CAD build for the part. Positions are in the model's coordinates, mm. Face numbers are marked on the shaded views. A direction names the side the tool comes from. Round coordinates to 2 decimals unless told otherwise and drop trailing zeros. Loops run counter-clockwise (first coordinate to the right, second up) from the corner with the lowest first, then second, coordinate; pieces in that order, holes last. Notation, with made-up numbers: (85, 29) - (105, 29) arc R10 ccw to (105, 37) - close; hole circle Ø5 at (-17.5, 20.5). An arc over 180 degrees is marked (long way). One line per question, with ' | ' between items.
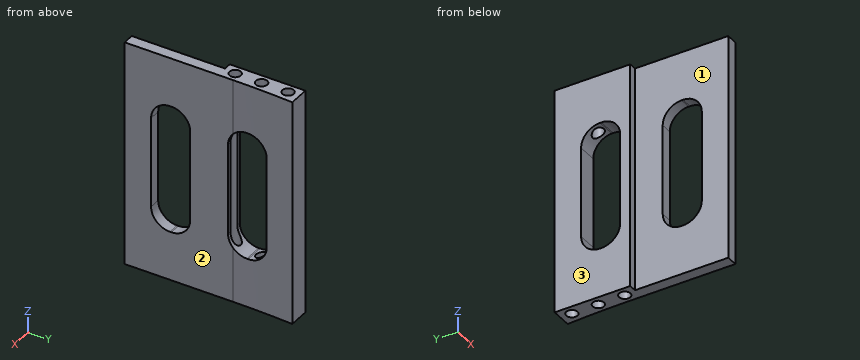
```python
from build123d import *

# Parameters (mm, degrees)
RESSALTO_EXTRUS_O1_DEPTH = 60
ESBO_O7_R                = 2.076684074
CORTE_EXTRUS_O5_DEPTH    = 61
ESBO_O8_W                = 84.528747457
ESBO_O8_H                = 37.806532702
CORTE_EXTRUS_O6_DEPTH    = 61
ESBO_O9_W                = 39.370764713
ESBO_O9_H                = 9.06161947
CORTE_EXTRUS_O7_DEPTH    = 61
ESBO_O10_W               = 32.42010131
ESBO_O10_H               = 62.029224545
CORTE_EXTRUS_O8_DEPTH    = 61
ESBO_O12_W               = 17.69499929
ESBO_O12_H               = 9
CORTE_EXTRUS_O10_DEPTH   = 61
ESBO_O13_W               = 2
ESBO_O13_H               = 24.699383264
CORTE_EXTRUS_O11_DEPTH   = 61
CORTE_EXTRUS_O12_DEPTH   = 6.517415369
ESBO_O15_R               = 1.5
CORTE_EXTRUS_O13_DEPTH   = 61.0000001


with BuildPart() as part:
    # Esboço1 → Ressalto-extrusão1 (new body)
    with BuildSketch(Plane.XY):
        with BuildLine():
            Line((13.569146061, 27.715579822), (13.569146061, 56.338894978))
            ThreePointArc((13.569146061, 56.338894978), (13.884544414, 68.892766914), (14.829943665, 81.414963086))
            ThreePointArc((14.829943665, 81.414963086), (11.193742071, 116.066691762), (-16.576524471, 95.024435265))
            Line((-16.576524471, 95.024435265), (-16.487894969, 94.437265709))
            Line((-16.487894969, 94.437265709), (-16.369382775, 93.652123615))
            ThreePointArc((-16.369382775, 93.652123615), (-14.270188159, 75.047972701), (-13.569146061, 56.338894978))
            Line((-13.569146061, 56.338894978), (-13.569146061, 27.715579822))
            ThreePointArc((-13.569146061, 27.715579822), (0, 21.02683783), (13.569146061, 27.715579822))
        make_face()
    extrude(amount=RESSALTO_EXTRUS_O1_DEPTH)

    # Esboço7 → Corte-extrusão5 (cut, through all)
    with BuildSketch(Plane(origin=(0, 0, 0), x_dir=(-1, 0, 0), z_dir=(0, 0, -1))):
        with Locations((-0.267564972, 95.19)):
            Circle(ESBO_O7_R)
    extrude(amount=-CORTE_EXTRUS_O5_DEPTH, mode=Mode.SUBTRACT)

    # Esboço8 → Corte-extrusão6 (cut, through all)
    with BuildSketch(Plane.XY.offset(60)):
        with Locations((-3.694100087, 100.318229437)):
            Rectangle(ESBO_O8_W, ESBO_O8_H)
    extrude(amount=-CORTE_EXTRUS_O6_DEPTH, mode=Mode.SUBTRACT)

    # Esboço9 → Corte-extrusão7 (cut, through all)
    with BuildSketch(Plane.XY.offset(60)):
        with Locations((-6.116236296, 23.184770087)):
            Rectangle(ESBO_O9_W, ESBO_O9_H)
    extrude(amount=-CORTE_EXTRUS_O7_DEPTH, mode=Mode.SUBTRACT)

    # Esboço10 → Corte-extrusão8 (cut, through all)
    with BuildSketch(Plane.XY.offset(60)):
        with Locations((-7.640904594, 58.730192094)):
            Rectangle(ESBO_O10_W, ESBO_O10_H)
    extrude(amount=-CORTE_EXTRUS_O8_DEPTH, mode=Mode.SUBTRACT)

    # Esboço12 → Corte-extrusão10 (cut, through all)
    with BuildSketch(Plane.XY.offset(60)):
        with Locations((10.676364632, 76.914963086)):
            Rectangle(ESBO_O12_W, ESBO_O12_H)
    extrude(amount=-CORTE_EXTRUS_O10_DEPTH, mode=Mode.SUBTRACT)

    # Esboço13 → Corte-extrusão11 (cut, through all)
    with BuildSketch(Plane.XY.offset(60)):
        with Locations((9.569146061, 40.065271454)):
            Rectangle(ESBO_O13_W, ESBO_O13_H)
    extrude(amount=-CORTE_EXTRUS_O11_DEPTH, mode=Mode.SUBTRACT)

    # Esboço14 → Corte-extrusão12 (cut, through all)
    with BuildSketch(Plane.ZY.offset(-8.569146061)):
        with BuildLine():
            Line((42, 55.065579822), (18, 55.065579822))
            ThreePointArc((18, 55.065579822), (14.464466094, 56.530045916), (13, 60.065579822))
            Line((13, 60.065579822), (13, 60.414963086))
            ThreePointArc((13, 60.414963086), (14.464466094, 63.950496992), (18, 65.414963086))
            Line((18, 65.414963086), (42, 65.414963086))
            ThreePointArc((42, 65.414963086), (45.535533906, 63.950496992), (47, 60.414963086))
            Line((47, 60.414963086), (47, 60.065579822))
            ThreePointArc((47, 60.065579822), (45.535533906, 56.530045916), (42, 55.065579822))
        make_face()
        with BuildLine():
            Line((42, 34.715579822), (18, 34.715579822))
            ThreePointArc((18, 34.715579822), (14.464466094, 36.180045916), (13, 39.715579822))
            Line((13, 39.715579822), (13, 40.065579822))
            ThreePointArc((13, 40.065579822), (14.464466094, 43.601113728), (18, 45.065579822))
            Line((18, 45.065579822), (42, 45.065579822))
            ThreePointArc((42, 45.065579822), (45.535533906, 43.601113728), (47, 40.065579822))
            Line((47, 40.065579822), (47, 39.715579822))
            ThreePointArc((47, 39.715579822), (45.535533906, 36.180045916), (42, 34.715579822))
        make_face()
    extrude(amount=-CORTE_EXTRUS_O12_DEPTH, mode=Mode.SUBTRACT)

    # Esboço15 → Corte-extrusão13 (cut, through all)
    with BuildSketch(Plane.XY.offset(60)):
        with Locations((11.069146061, 69.414963086)):
            Circle(ESBO_O15_R)
        with Locations((11.069146061, 62.414963086)):
            Circle(ESBO_O15_R)
        with Locations((11.069146061, 55.414963086)):
            Circle(ESBO_O15_R)
    extrude(amount=-CORTE_EXTRUS_O13_DEPTH, mode=Mode.SUBTRACT)


solid = part.part
```
(1) Cut at D-D, the plane x = 11.45. State how many separate pieces and enclosed holes the cut face has, then the cut area to 3 significant figures.
Results found:
separate pieces: 5 | enclosed holes: 1 | area: 1,650 mm²
(2) Cut at C-C, the plane z = 7. Write the cut outline in (x, y).
Results found:
outline: (8.57, 52.41) - (10.57, 52.41) - (10.57, 27.72) - (13.57, 27.72) - (13.57, 56.34) arc R250 cw to (14.09, 72.41) - (8.57, 72.41) - close; hole circle Ø3 at (11.07, 55.41); hole circle Ø3 at (11.07, 62.41); hole circle Ø3 at (11.07, 69.41)
(3) Cut at B-B, the plane y = 43. Write the cut outline in (x, z), then the cut area to 3 significant figures.
Results found:
outline: (10.57, 0) - (13.57, 0) - (13.57, 13.95) - (10.57, 13.95) - close; (10.57, 46.05) - (13.57, 46.05) - (13.57, 60) - (10.57, 60) - close | area: 83.7 mm²
(4) Cut at A-A, the plane z = 15.5. Write the cut outline in (x, y).
Results found:
outline: (8.57, 52.41) - (10.57, 52.41) - (10.57, 44.4) - (13.57, 44.4) - (13.57, 55.74) - (12.53, 55.74) arc R1.5 cw (long way) to (9.6, 55.74) - (8.57, 55.74) - close; (8.57, 64.75) - (13.71, 64.75) arc R250 cw to (14.09, 72.41) - (8.57, 72.41) - close; (10.57, 27.72) - (13.57, 27.72) - (13.57, 35.39) - (10.57, 35.39) - close; hole circle Ø3 at (11.07, 69.41)
(5) Tool access for the marked faces 1, 2 and 3: list every direction of +Z, -Z, +X, -X, +Y, -Y with a clear straight run to the whole face (end or side of a thin tool).
Results found:
face 1: +Z, -Z, -X, -Y | face 2: +Z, -Z, +X, -Y | face 3: +Z, -Z, -X, +Y, -Y
(6) Drop flat-ended pins along their axis: P1, Ø1.8, axis at x = 11.07, y = 62.41, coming from the +Z side; P2, Ø4, axis at y = 36, z = 36.5, coming from the -X side; P3, Ø0.6, axis at x = 10, z = 39.5, coming from the -Y side. Give the stop position or say it passes through.
Results found:
P1: passes through | P2: stops at x = 10.57 | P3: stops at y = 52.41
(7) Probe L1, parallel to Y at x = 11.5, z = 54.5; L2, parallel to Y at x = 10.7, z = 20; L3, parallel to X at y = 65.5, z = 42. List the from-to ranges inside material, lowest first.
Results found:
L1: y = 27.72 to 53.98, 56.85 to 60.98, 63.85 to 67.98, 70.85 to 72.41 | L2: y = 27.72 to 34.72, 45.07 to 53.96, 65.41 to 67.96, 70.87 to 72.41 | L3: x = 8.57 to 13.74
